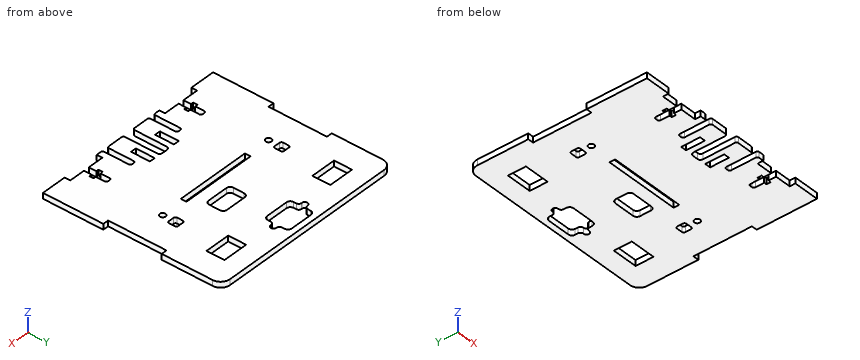
from build123d import *

# Parameters (mm, degrees)
ESBO_O1_W                = 100
ESBO_O1_H                = 95
RESSALTO_EXTRUS_O1_DEPTH = 1.5
ESBO_O3_W                = 3
ESBO_O3_H                = 32
RESSALTO_EXTRUS_O2_DEPTH = 3
ESBO_O2_R                = 1.5
ESBO_O2_W                = 40
ESBO_O2_H                = 3
CORTE_EXTRUS_O1_DEPTH    = 72.233770081
CUT_EXTRUDE3_DEPTH       = 72.233770081
CUT_EXTRUDE3_DEPTH_BACK  = 72.233770081
CUT_EXTRUDE5_DEPTH       = 72.186375101
CUT_EXTRUDE5_DEPTH_BACK  = 72.186375101
CUT_EXTRUDE6_DEPTH       = 72.186375101
CUT_EXTRUDE6_DEPTH_BACK  = 72.186375101
SKETCH7_W                = 13.5
SKETCH7_H                = 9.5
CUT_EXTRUDE7_DEPTH       = 72.186375101
CUT_EXTRUDE7_DEPTH_BACK  = 72.186375101
SKETCH8_W                = 3
SKETCH8_H                = 10
CUT_EXTRUDE8_DEPTH       = 72.186375101
CUT_EXTRUDE8_DEPTH_BACK  = 72.186375101
CUT_EXTRUDE10_DEPTH      = 72.186375101
CUT_EXTRUDE10_DEPTH_BACK = 72.186375101
CUT_EXTRUDE11_DEPTH      = 72.186375101
CUT_EXTRUDE11_DEPTH_BACK = 72.186375101
FILLET1_R                = 1
FILLET2_R                = 5


with BuildPart() as part:
    # Esboço1 → Ressalto-extrusão1 (new, symmetric)
    with BuildSketch(Plane.XY):
        Rectangle(ESBO_O1_W, ESBO_O1_H)
    extrude(amount=RESSALTO_EXTRUS_O1_DEPTH, both=True)

    # Esboço3 → Ressalto-extrusão2 (add, through all)
    with BuildSketch(Plane.XY.offset(1.5)):
        with Locations((-51.5, 31.5)):
            Rectangle(ESBO_O3_W, ESBO_O3_H)
        with Locations((-51.5, -31.5)):
            Rectangle(ESBO_O3_W, ESBO_O3_H)
        with Locations((51.5, -31.5)):
            Rectangle(ESBO_O3_W, ESBO_O3_H)
        with Locations((51.5, 31.5)):
            Rectangle(ESBO_O3_W, ESBO_O3_H)
    extrude(amount=-RESSALTO_EXTRUS_O2_DEPTH)

    # Esboço2 → Corte-extrusão1 (cut, through all)
    with BuildSketch(Plane.XY.offset(1.5)):
        with Locations((-33, -1)):
            Circle(ESBO_O2_R)
        with Locations(Location((33, -1, 0), (0, 0, 180))):
            Circle(ESBO_O2_R)
        with Locations((0, -1)):
            Rectangle(ESBO_O2_W, ESBO_O2_H)
    extrude(amount=-CORTE_EXTRUS_O1_DEPTH, mode=Mode.SUBTRACT)

    # Sketch4 → Cut-Extrude3 (cut, two sides: drawn at the far end of the back side and taken through both)
    with BuildSketch(Plane.XY.offset(1.5).offset(-CUT_EXTRUDE3_DEPTH_BACK)):
        with BuildLine():
            Line((-34.5, 8.5), (-31.5, 8.5))
            ThreePointArc((-31.5, 8.5), (-30.792893219, 8.207106781), (-30.5, 7.5))
            Line((-30.5, 7.5), (-30.5, 4.5))
            ThreePointArc((-30.5, 4.5), (-30.792893219, 3.792893219), (-31.5, 3.5))
            Line((-31.5, 3.5), (-34.5, 3.5))
            ThreePointArc((-34.5, 3.5), (-35.207106781, 3.792893219), (-35.5, 4.5))
            Line((-35.5, 4.5), (-35.5, 7.5))
            ThreePointArc((-35.5, 7.5), (-35.207106781, 8.207106781), (-34.5, 8.5))
        make_face()
        with BuildLine():
            Line((30.5, 7.5), (30.5, 4.5))
            ThreePointArc((30.5, 4.5), (30.792893219, 3.792893219), (31.5, 3.5))
            Line((31.5, 3.5), (34.5, 3.5))
            ThreePointArc((34.5, 3.5), (35.207106781, 3.792893219), (35.5, 4.5))
            Line((35.5, 4.5), (35.5, 7.5))
            ThreePointArc((35.5, 7.5), (35.207106781, 8.207106781), (34.5, 8.5))
            Line((34.5, 8.5), (31.5, 8.5))
            ThreePointArc((31.5, 8.5), (30.792893219, 8.207106781), (30.5, 7.5))
        make_face()
    extrude(amount=CUT_EXTRUDE3_DEPTH + CUT_EXTRUDE3_DEPTH_BACK, mode=Mode.SUBTRACT)

    # Sketch6 → Cut-Extrude5 (cut, two sides: drawn at the far end of the back side and taken through both)
    with BuildSketch(Plane.XY.offset(-CUT_EXTRUDE5_DEPTH_BACK)):
        with BuildLine():
            Line((-6, 44.5), (6, 44.5))
            ThreePointArc((6, 44.5), (7.414213562, 43.914213562), (8, 42.5))
            Line((8, 42.5), (8, 41))
            ThreePointArc((8, 41), (8.439339828, 39.939339828), (9.5, 39.5))
            Line((9.5, 39.5), (9.75, 39.5))
            ThreePointArc((9.75, 39.5), (11.25, 38), (9.75, 36.5))
            Line((9.75, 36.5), (9.5, 36.5))
            ThreePointArc((9.5, 36.5), (8.439339828, 36.060660172), (8, 35))
            Line((8, 35), (8, 33.5))
            ThreePointArc((8, 33.5), (7.414213562, 32.085786438), (6, 31.5))
            Line((6, 31.5), (-6, 31.5))
            ThreePointArc((-6, 31.5), (-7.414213562, 32.085786438), (-8, 33.5))
            Line((-8, 33.5), (-8, 35))
            ThreePointArc((-8, 35), (-8.439339828, 36.060660172), (-9.5, 36.5))
            Line((-9.5, 36.5), (-9.75, 36.5))
            ThreePointArc((-9.75, 36.5), (-11.25, 38), (-9.75, 39.5))
            Line((-9.75, 39.5), (-9.5, 39.5))
            ThreePointArc((-9.5, 39.5), (-8.439339828, 39.939339828), (-8, 41))
            Line((-8, 41), (-8, 42.5))
            ThreePointArc((-8, 42.5), (-7.414213562, 43.914213562), (-6, 44.5))
        make_face()
    extrude(amount=CUT_EXTRUDE5_DEPTH + CUT_EXTRUDE5_DEPTH_BACK, mode=Mode.SUBTRACT)

    # Sketch7 → Cut-Extrude6 (cut, two sides: drawn at the far end of the back side and taken through both)
    with BuildSketch(Plane.XY.offset(-CUT_EXTRUDE6_DEPTH_BACK)):
        with Locations((-33, 32.75)):
            Rectangle(SKETCH7_W, SKETCH7_H)
        with Locations((33, 32.75)):
            Rectangle(SKETCH7_W, SKETCH7_H)
    extrude(amount=CUT_EXTRUDE6_DEPTH + CUT_EXTRUDE6_DEPTH_BACK, mode=Mode.SUBTRACT)

    # Sketch8 → Cut-Extrude7 (cut, two sides: drawn at the far end of the back side and taken through both)
    with BuildSketch(Plane.XY.offset(-CUT_EXTRUDE7_DEPTH_BACK)):
        with Locations((-7.5, -33.23)):
            Rectangle(SKETCH8_W, SKETCH8_H)
        with Locations((7.5, -33.23)):
            Rectangle(SKETCH8_W, SKETCH8_H)
    extrude(amount=CUT_EXTRUDE7_DEPTH + CUT_EXTRUDE7_DEPTH_BACK, mode=Mode.SUBTRACT)

    # Sketch9 → Cut-Extrude8 (cut, two sides: drawn at the far end of the back side and taken through both)
    with BuildSketch(Plane.XY.offset(-CUT_EXTRUDE8_DEPTH_BACK)):
        with BuildLine():
            Line((2.5, 16.5), (13.5, 16.5))
            ThreePointArc((13.5, 16.5), (14.914213562, 15.914213562), (15.5, 14.5))
            Line((15.5, 14.5), (15.5, 8.8))
            ThreePointArc((15.5, 8.8), (14.914213562, 7.385786438), (13.5, 6.8))
            Line((13.5, 6.8), (2.5, 6.8))
            ThreePointArc((2.5, 6.8), (1.085786438, 7.385786438), (0.5, 8.8))
            Line((0.5, 8.8), (0.5, 14.5))
            ThreePointArc((0.5, 14.5), (1.085786438, 15.914213562), (2.5, 16.5))
        make_face()
    extrude(amount=CUT_EXTRUDE8_DEPTH + CUT_EXTRUDE8_DEPTH_BACK, mode=Mode.SUBTRACT)

    # Sketch11 → Cut-Extrude10 (cut, two sides: drawn at the far end of the back side and taken through both)
    with BuildSketch(Plane.XY.offset(-CUT_EXTRUDE10_DEPTH_BACK)):
        with BuildLine():
            Line((13, -33.5), (13, -47.5))
            Line((13, -47.5), (16, -47.5))
            Line((16, -47.5), (16, -33.5))
            ThreePointArc((16, -33.5), (15.707106781, -32.792893219), (15, -32.5))
            Line((15, -32.5), (14, -32.5))
            ThreePointArc((14, -32.5), (13.292893219, -32.792893219), (13, -33.5))
        make_face()
        with BuildLine():
            Line((-1.5, -28), (1.5, -28))
            ThreePointArc((1.5, -28), (2.560660172, -28.439339828), (3, -29.5))
            Line((3, -29.5), (3, -47.5))
            Line((3, -47.5), (-3, -47.5))
            Line((-3, -47.5), (-3, -29.5))
            ThreePointArc((-3, -29.5), (-2.560660172, -28.439339828), (-1.5, -28))
        make_face()
        with BuildLine():
            Line((-15, -32.5), (-14, -32.5))
            ThreePointArc((-14, -32.5), (-13.292893219, -32.792893219), (-13, -33.5))
            Line((-13, -33.5), (-13, -47.5))
            Line((-13, -47.5), (-16, -47.5))
            Line((-16, -47.5), (-16, -33.5))
            ThreePointArc((-16, -33.5), (-15.707106781, -32.792893219), (-15, -32.5))
        make_face()
    extrude(amount=CUT_EXTRUDE10_DEPTH + CUT_EXTRUDE10_DEPTH_BACK, mode=Mode.SUBTRACT)

    # Sketch12 → Cut-Extrude11 (cut, two sides: drawn at the far end of the back side and taken through both)
    with BuildSketch(Plane.XY.offset(-CUT_EXTRUDE11_DEPTH_BACK)):
        with BuildLine():
            Line((-39.5, -47.5), (-19.5, -47.5))
            Line((-19.5, -47.5), (-19.5, -44.5))
            Line((-19.5, -44.5), (-28, -44.5))
            Line((-28, -44.5), (-28, -40.5))
            Line((-28, -40.5), (-26.65, -40.5))
            Line((-26.65, -40.5), (-26.65, -38.23))
            Line((-26.65, -38.23), (-28, -38.23))
            Line((-28, -38.23), (-28, -33.5))
            ThreePointArc((-28, -33.5), (-28.292893219, -32.792893219), (-29, -32.5))
            Line((-29, -32.5), (-30, -32.5))
            ThreePointArc((-30, -32.5), (-30.707106781, -32.792893219), (-31, -33.5))
            Line((-31, -33.5), (-31, -38.23))
            Line((-31, -38.23), (-32.35, -38.23))
            Line((-32.35, -38.23), (-32.35, -40.5))
            Line((-32.35, -40.5), (-31, -40.5))
            Line((-31, -40.5), (-31, -44.5))
            Line((-31, -44.5), (-39.5, -44.5))
            Line((-39.5, -44.5), (-39.5, -47.5))
        make_face()
        with BuildLine():
            Line((28, -38.23), (28, -33.5))
            ThreePointArc((28, -33.5), (28.292893219, -32.792893219), (29, -32.5))
            Line((29, -32.5), (30, -32.5))
            ThreePointArc((30, -32.5), (30.707106781, -32.792893219), (31, -33.5))
            Line((31, -33.5), (31, -38.23))
            Line((31, -38.23), (32.35, -38.23))
            Line((32.35, -38.23), (32.35, -40.5))
            Line((32.35, -40.5), (31, -40.5))
            Line((31, -40.5), (31, -44.5))
            Line((31, -44.5), (39.5, -44.5))
            Line((39.5, -44.5), (39.5, -47.5))
            Line((39.5, -47.5), (19.5, -47.5))
            Line((19.5, -47.5), (19.5, -44.5))
            Line((19.5, -44.5), (28, -44.5))
            Line((28, -44.5), (28, -40.5))
            Line((28, -40.5), (26.65, -40.5))
            Line((26.65, -40.5), (26.65, -38.23))
            Line((26.65, -38.23), (28, -38.23))
        make_face()
    extrude(amount=CUT_EXTRUDE11_DEPTH + CUT_EXTRUDE11_DEPTH_BACK, mode=Mode.SUBTRACT)

    # Fillet1
    fillet1_edges = [part.edges().sort_by_distance(p)[0] for p in [
        (16, -47.5, 0),
        (13, -47.5, 0),
        (-13, -47.5, 0),
        (-16, -47.5, 0),
        (3, -47.5, 0),
        (-3, -47.5, 0),
    ]]
    fillet(fillet1_edges, radius=FILLET1_R)

    # Fillet2
    fillet2_edges = [part.edges().sort_by_distance(p)[0] for p in [
        (-53, 47.5, 0),
        (53, 47.5, 0),
    ]]
    fillet(fillet2_edges, radius=FILLET2_R)


solid = part.part
Build history of the part. All positions in model axes, mm. Give positions to 0.01 mm unless a question says otherwise; leave off trailing zeros. Order: outer loops, then holes, each group sorted by start corner. A loop starts at its lowest first (then second) coordinate and runs counter-clockwise, first axis right, second up. Notation, with made-up numbers: M 61.5,81.5 L 93.5,81.5 A10 cw 93.5,98.5 Z; hole C 40.5,14.25 d1. An arc over 180 degrees is marked long. Put each result on its own line as item: value.
Item 1: Flat gauge pins, fed straight in: pin 1 Ø2.5 at (x, y) = (33, -1) entering from +Z; pin 2 Ø0.9 at (y, z) = (5.5, 0) entering from +X. Where does each tip first touch, or does it go through?
From the geometry:
pin 1: passes through
pin 2: stops at x = 50
Item 2: Slice it at A-A, the plane y = -1. Write the cut outline in (x, z), plus the area to 3 significant figures.
From the geometry:
outline: M -50,-1.5 L -34.5,-1.5 L -34.5,1.5 L -50,1.5 Z; M -31.5,-1.5 L -20,-1.5 L -20,1.5 L -31.5,1.5 Z; M 20,-1.5 L 31.5,-1.5 L 31.5,1.5 L 20,1.5 Z; M 34.5,-1.5 L 50,-1.5 L 50,1.5 L 34.5,1.5 Z
area: 162 mm2
Item 3: Slice it at C-C, the plane y = -12. Write the cut outline in (x, z), plus the area to 3 significant figures.
From the geometry:
outline: M -50,-1.5 L 50,-1.5 L 50,1.5 L -50,1.5 Z
area: 300 mm2
Item 4: Probe line 1 (Y direction, x = -33, z = -0.75); line 2 (X direction, y = -31.5, z = 0.9); line 3 (X direction, y = 33, z = -0.35). List the from-to ranges inside material, lowest first. Write a range as [from, to].
From the geometry:
line 1: y = [-44.5, -2.5], [0.5, 3.5], [8.5, 28], [37.5, 47.5]
line 2: x = [-53, -9], [-6, -3], [3, 6], [9, 53]
line 3: x = [-53, -39.75], [-26.25, -7.94], [7.94, 26.25], [39.75, 53]
Item 5: Slice it at B-B, the plane z = 0.2. Give the number of separate pieces and of enclosed holes in the cut face, plus the area to 3 significant figures.
From the geometry:
separate pieces: 1
enclosed holes: 11
area: 8,600 mm2
